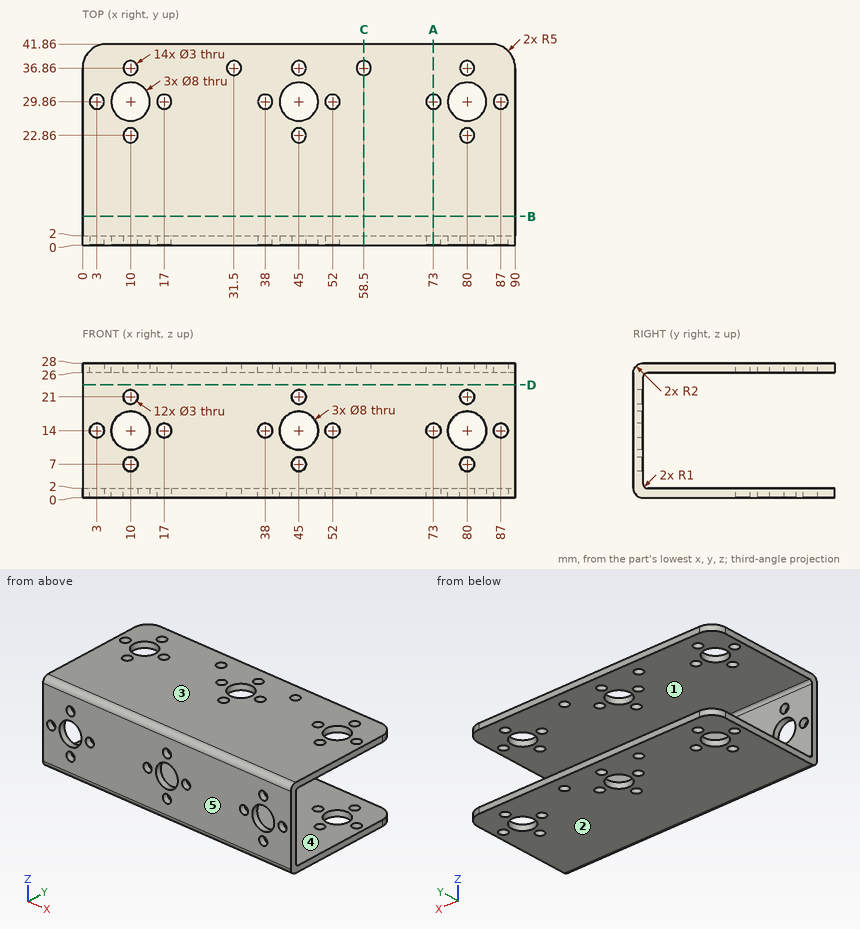
The figure shows three views and two pictorial views of one solid part (mm, origin at its lowest corner). Answer the questions. A direction names the side the tool comes from. Round coordinates to 2 decimals unless told otherwise and drop trailing zeros. Loops run counter-clockwise (first coordinate to the right, second up) from the corner with the lowest first, then second, coordinate; pieces in that order, holes last. Notation, with made-up numbers: (-31.5, 17) -> (1.5, 17) arc R35 ccw to (1.5, 49) -> close; hole circle Ø4 at (78.25, 5.5). An arc over 180 degrees is marked (long way). Use one line per item in the form item = value.
(1) Find section A-A on x = 73. Give the vertices of the cut face in (y, z), then the cut area to 3 significant figures.
Answer list:
outline = (0, 2) arc R2 ccw to (2, 0) -> (28.36, 0) -> (28.36, 2) -> (3, 2) arc R1 cw to (2, 3) -> (2, 12.5) -> (0, 12.5) -> close; (0, 15.5) -> (2, 15.5) -> (2, 25) arc R1 cw to (3, 26) -> (28.36, 26) -> (28.36, 28) -> (2, 28) arc R2 ccw to (0, 26) -> close; (31.36, 0) -> (41.86, 0) -> (41.86, 2) -> (31.36, 2) -> close; (31.36, 26) -> (41.86, 26) -> (41.86, 28) -> (31.36, 28) -> close
area = 196 mm2
(2) A tool of negligible diameter and unlimited length cuts with its end or side. For the marked faces 1 and 2, from which of +Z, -Z, +X, -X, +Y, -Y can it reach the whole face along a straight path? Write none if from no direction.
Answer list:
face_1 = +X, -X, +Y
face_2 = -Z, +X, -X, +Y, -Y
(3) For a pull along Z with two mould halves and no side action, classify the marked faces 3, 4 and 5 as released by +Z, released by -Z, zero draft, split by the parting line, or undercut.
Answer list:
face_3 = released by +Z
face_4 = undercut
face_5 = zero draft
(4) Find section C-C on x = 58.5. Give the vertices of the cut face in (y, z).
Answer list:
outline = (0, 2) arc R2 ccw to (2, 0) -> (35.36, 0) -> (35.36, 2) -> (3, 2) arc R1 cw to (2, 3) -> (2, 25) arc R1 cw to (3, 26) -> (35.36, 26) -> (35.36, 28) -> (2, 28) arc R2 ccw to (0, 26) -> close; (38.36, 0) -> (41.86, 0) -> (41.86, 2) -> (38.36, 2) -> close; (38.36, 26) -> (41.86, 26) -> (41.86, 28) -> (38.36, 28) -> close
(5) Straight lines are drawn through the part: line 1 (X direction, y = 1.45, z = 7); line 2 (Z direction, x = 38.5, y = 38); line 3 (Y direction, x = 10, z = 26.8). For each, find the intervals that lie inside material, in ascending order.
Answer list:
line_1 = 0 to 8.5, 11.5 to 43.5, 46.5 to 78.5, 81.5 to 90
line_2 = 0 to 2, 26 to 28
line_3 = 0.17 to 21.36, 24.36 to 25.86, 33.86 to 35.36, 38.36 to 41.86
(6) Find section B-B on y = 6. Give the vertices of the cut face in (x, z).
Answer list:
outline = (0, 0) -> (90, 0) -> (90, 2) -> (0, 2) -> close; (0, 26) -> (90, 26) -> (90, 28) -> (0, 28) -> close
(7) Find section D-D on z = 23.5. Give the vertices of the cut face in (x, y).
Answer list:
outline = (0, 0) -> (90, 0) -> (90, 2) -> (0, 2) -> close
(8) Flat-ended cylindrical pins translate along their axes: P1, Ø2.5, axis at x = 45, y = 22.86, coming from the -Z side; P2, Ø8, axis at x = 13, z = 18.5, coming from the +Y side. Find the tip coordinate at first contact, or state that the pin passes through.
Answer list:
P1 = through
P2 = 2
